```python
from build123d import *

# Parameters (mm, degrees)
F2_DEPTH      = 1.2
F3_DEPTH      = 1.201
F3_DEPTH_BACK = 1.201
F4_R          = 1.6
F5_R          = 3


with BuildPart() as f2:
    # F0 (on Right) → F2 (new body, symmetric)
    with BuildSketch(Plane.YZ):
        Polygon((6.7, 3.6), (-6.7, 3.6), (-6.7, 1), (-4.8, 1), (-4.8, -29), (4.8, -29), (4.8, 1), (6.7, 1), align=None)
    extrude(amount=F2_DEPTH, both=True)

    # F1 (on Right) → F3 (cut, two sides)
    with BuildSketch(Plane.YZ) as f3_sk:
        with BuildLine():
            Line((1.8, -7.4), (1.8, -1.4))
            ThreePointArc((1.8, -1.4), (0, 0.4), (-1.8, -1.4))
            Line((-1.8, -1.4), (-1.8, -7.4))
            ThreePointArc((-1.8, -7.4), (0, -9.2), (1.8, -7.4))
        make_face()
        with BuildLine():
            Line((1.8, -25.4), (1.8, -19.4))
            ThreePointArc((1.8, -19.4), (0, -17.6), (-1.8, -19.4))
            Line((-1.8, -19.4), (-1.8, -25.4))
            ThreePointArc((-1.8, -25.4), (0, -27.2), (1.8, -25.4))
        make_face()
    extrude(amount=-F3_DEPTH, mode=Mode.SUBTRACT)
    extrude(f3_sk.sketch, amount=F3_DEPTH_BACK, mode=Mode.SUBTRACT)

    # F4
    f4_edges = [f2.edges().sort_by_distance(p)[0] for p in [
        (0, 6.7, 3.6),
        (0, -6.7, 3.6),
    ]]
    fillet(f4_edges, radius=F4_R)

    # F5
    f5_edges = [f2.edges().sort_by_distance(p)[0] for p in [
        (0, 4.8, -29),
        (0, -4.8, -29),
    ]]
    fillet(f5_edges, radius=F5_R)


solid = f2.part
```
Geometry check sheet. Reference: the model listing, model coordinates, mm. A direction names the side the tool comes from. Coordinates: 2 decimals unless noted, no trailing zeros. Write each loop counter-clockwise with the first axis right and the second up, starting at its lowest first coordinate (ties: lowest second). Pieces come first, ordered by that corner, then holes. Notation, with made-up numbers: M 73.5,63.25 L 90.5,63.25 A26 ccw 90.5,80.25 Z; hole C 79.25,2 d1. An arc over 180 degrees is marked long. Use one line per item in the form item = value. Start each with the question number.
1) Section check A-A on y = 0. Enter the section's corners in (x, z).
2) Release check for a two-part mould opening along Y. For faces 1 (the flat face through (-1.2, 0, -12)), 2 (the flat face through (0, 6.7, 1.5)), 3 (the cylindrical face through (0, 0, -27.2)), 4 (the flat face through (0, -4.8, -12)) record: pulls with the +Y half, pulls with the -Y half, needs draft (parallel to the pull), parting line crosses it, or undercut.
3) Section check C-C on z = -5. Enter the section's corners in (x, y).
4) Section check B-B on x = -0.25. Enter the section's corners in (y, z), and give its area (3 significant figures).
5) Go/stop test with flat-tipped pins: pin 1 Ø1.2 at (x, z) = (0, -19) entering from +Y; pin 2 Ø0.7 at (x, z) = (0, -4) entering from -Y. Record where each tip stops, or that it passes through.
6) Section check D-D on z = -10.5. Enter the section's corners in (x, y).
7) Set-up check for faces 5 (the flat face through (1.2, 0, -12)), 6 (the flat face through (0, -1.8, -22)), 7 (the cylindrical face through (0.02, -6.22, 3.14)), 8 (the flat face through (0, 4.8, -13)), 9 (the flat face through (0, -6, 1)): record each of +Z, -Z, +X, -X, +Y, -Y from which the full face is reachable in a straight line by a thin tool's end or side.
8) Thickness scan on probe 1 along Y at (x, z) = (-0.35, -20); probe 2 along Z at (x, y) = (-0.55, 1.25); probe 3 along Z at (x, y) = (-0.7, -2). Record the ranges inside material, lowest first. Write a range as from..to.
Responses:
q1.outline = M -1.2,-29 L 1.2,-29 L 1.2,-27.2 L -1.2,-27.2 Z; M -1.2,-17.6 L 1.2,-17.6 L 1.2,-9.2 L -1.2,-9.2 Z; M -1.2,0.4 L 1.2,0.4 L 1.2,3.6 L -1.2,3.6 Z
q2.face_1 = needs draft
q2.face_2 = pulls with the +Y half
q2.face_3 = undercut
q2.face_4 = pulls with the -Y half
q3.outline = M -1.2,-4.8 L 1.2,-4.8 L 1.2,-1.8 L -1.2,-1.8 Z; M -1.2,1.8 L 1.2,1.8 L 1.2,4.8 L -1.2,4.8 Z
q4.outline = M -6.7,1 L -4.8,1 L -4.8,-26 A3 ccw -1.8,-29 L 1.8,-29 A3 ccw 4.8,-26 L 4.8,1 L 6.7,1 L 6.7,2 A1.6 ccw 5.1,3.6 L -5.1,3.6 A1.6 ccw -6.7,2 Z; hole M -1.8,-25.4 A1.8 ccw 1.8,-25.4 L 1.8,-19.4 A1.8 ccw -1.8,-19.4 Z; hole M -1.8,-7.4 A1.8 ccw 1.8,-7.4 L 1.8,-1.4 A1.8 ccw -1.8,-1.4 Z
q4.area = 254 mm2
q5.pin_1 = 4.8
q5.pin_2 = -4.8
q6.outline = M -1.2,-4.8 L 1.2,-4.8 L 1.2,4.8 L -1.2,4.8 Z
q7.face_5 = +Z, -Z, +X, +Y, -Y
q7.face_6 = +X, -X
q7.face_7 = +Z, +X, -X, -Y
q7.face_8 = -Z, +X, -X, +Y
q7.face_9 = -Z, +X, -X, -Y
q8.probe_1 = -4.8..-1.8, 1.8..4.8
q8.probe_2 = -29..-26.7, -18.1..-8.7, -0.1..3.6
q8.probe_3 = -28.99..3.6
